Check sheet for the modelled part. Datum: model origin and axes. Units: mm. A direction names the side the tool comes from. Give positions to 0.01 mm unless a question says otherwise; leave off trailing zeros. Loops run counter-clockwise (first coordinate to the right, second up) from the corner with the lowest first, then second, coordinate; pieces in that order, holes last. Notation, with made-up numbers: (28.25, 51.5) - (37.25, 51.5) arc R7 ccw to (37.25, 59.5) - close; hole circle Ø9 at (67.5, -13.75). An arc over 180 degrees is marked (long way). Answer in a Markdown table with one row per item. Add a question column.
(1) Thickness scan on L1, parallel to Z at x = 0.75, y = 2.75; L2, parallel to Z at x = 2.5, y = 2.5; L3, parallel to Z at x = 0.25, y = -2.75. Record the ranges inside material, lowest first.
(2) Sectioned sample at A-A on z = 14. Enter the section's corners in (x, y) (1 decimal), then the cut area to 3 significant figures.
(3) Go/stop test with flat-tipped pins: P1, Ø4, axis at y = -2, z = 27, coming from the +X side; P2, Ø2, axis at x = 3, z = 17, coming from the -Y side; P3, Ø1, axis at x = 0, z = 12, coming from the +Y side; P4, Ø1, axis at y = -4, z = 27, coming from the -X side. Record where each tip stops, or that it passes through.
(4) Sectioned sample at B-B on y = 4.5. Enter the section's corners in (x, z).
(5) Set-up check for faces 1 (the face through (0, 0, 30.607)), 2 (the face through (2, 2, 3.302)): record each of +Z, -Z, +X, -X, +Y, -Y from which the full face is reachable in a straight line by a thin tool's end or side.
from build123d import *

# Parameters (mm, degrees)
SKETCH3_R           = 3.175
BOSS_EXTRUDE1_DEPTH = 3.302
CUT_SWEEP1_PITCH    = 1.27
SKETCH10_R          = 2.2225
BOSS_EXTRUDE5_DEPTH = 26.797
SKETCH9_R           = 5.08
BOSS_EXTRUDE4_DEPTH = 0.127
DOME3_FACE_RADIUS   = 5.08
DOME3_HEIGHT        = 2.38
SKETCH11_R          = 1.8415
BOSS_EXTRUDE6_DEPTH = 0.508


with BuildPart() as part:
    # Sketch3 → Boss-Extrude1 (new body)
    with BuildSketch(Plane.XY):
        with Locations(Location((0, 0, 0), (0, 0, 180))):
            Circle(SKETCH3_R)
    extrude(amount=BOSS_EXTRUDE1_DEPTH)

    # Cut-Sweep1: arcs per turn and ends read off the stored shape
    # Cut-Sweep1: the profile of Sketch5 profile screwed along a left-hand helix through 4.5 turns, 8 arcs to a turn; built about Z, then put on its axis
    cut_sweep1_z = Axis((0, 0, 0), (0, 0, 1))
    cut_sweep1_corners = [(2.54, 0, -1.397), (3.1753, 0, -1.763790626), (3.1753, 0, -0.776209374), (2.54, 0, -1.143)]
    with BuildLine(mode=Mode.PRIVATE) as cut_sweep1_profile:
        Line(cut_sweep1_corners[0], cut_sweep1_corners[1])
        Line(cut_sweep1_corners[1], cut_sweep1_corners[2])
        Line(cut_sweep1_corners[2], cut_sweep1_corners[3])
        Line(cut_sweep1_corners[3], cut_sweep1_corners[0])
    cut_sweep1_cap = Face(cut_sweep1_profile.wire())
    cut_sweep1_turn_angles = [0, -22.5, -45, -67.5, -90, -112.5, -135, -157.5, -180, -202.5, -225, -247.5, -270, -292.5, -315, -337.5, -360]
    cut_sweep1_turn_weights = [1, 0.9238795325112867, 1, 0.9238795325112867, 1, 0.9238795325112867, 1, 0.9238795325112867, 1, 0.9238795325112867, 1, 0.9238795325112867, 1, 0.9238795325112867, 1, 0.9238795325112867, 1]
    cut_sweep1_turn_rails = [Edge.make_bspline([Vector(p[0], p[1], 0).rotate(cut_sweep1_z, cut_sweep1_turn_angles[k]) / cut_sweep1_turn_weights[k] + Vector(0, 0, p[2] + -CUT_SWEEP1_PITCH * cut_sweep1_turn_angles[k] / 360) for k in range(17)], [0, 0, 0, 1, 1, 2, 2, 3, 3, 4, 4, 5, 5, 6, 6, 7, 7, 8, 8, 8], 2, cut_sweep1_turn_weights) for p in cut_sweep1_corners]
    cut_sweep1_turn_sides = [Face.make_surface_from_curves(cut_sweep1_turn_rails[p[0]], cut_sweep1_turn_rails[p[1]]) for p in [(0, 1), (1, 2), (2, 3), (3, 0)]]
    cut_sweep1_last_angles = [-1440, -1462.5, -1485, -1507.5, -1530, -1552.5, -1575, -1597.5, -1620]
    cut_sweep1_last_weights = [1, 0.9238795325112867, 1, 0.9238795325112867, 1, 0.9238795325112867, 1, 0.9238795325112867, 1]
    cut_sweep1_last_rails = [Edge.make_bspline([Vector(p[0], p[1], 0).rotate(cut_sweep1_z, cut_sweep1_last_angles[k]) / cut_sweep1_last_weights[k] + Vector(0, 0, p[2] + -CUT_SWEEP1_PITCH * cut_sweep1_last_angles[k] / 360) for k in range(9)], [0, 0, 0, 1, 1, 2, 2, 3, 3, 4, 4, 4], 2, cut_sweep1_last_weights) for p in cut_sweep1_corners]
    cut_sweep1_last_sides = [Face.make_surface_from_curves(cut_sweep1_last_rails[p[0]], cut_sweep1_last_rails[p[1]]) for p in [(0, 1), (1, 2), (2, 3), (3, 0)]]
    cut_sweep1 = Plane(origin=(0, 0, 0), x_dir=(0, 1, 0), z_dir=(0, 0, 1)) * Solid(Shell([*[p.moved(Location((0, 0, CUT_SWEEP1_PITCH * i))) for i in range(4) for p in cut_sweep1_turn_sides], *cut_sweep1_last_sides, cut_sweep1_cap, cut_sweep1_cap.rotate(cut_sweep1_z, -1620).moved(Location((0, 0, -CUT_SWEEP1_PITCH * -1620 / 360)))]))
    add(cut_sweep1, mode=Mode.SUBTRACT)

    # Sketch10 → Boss-Extrude5 (add)
    with BuildSketch(Plane.XY.offset(3.302)):
        Circle(SKETCH10_R)
    extrude(amount=BOSS_EXTRUDE5_DEPTH)

    # Sketch9 → Boss-Extrude4 (add)
    with BuildSketch(Plane.XY):
        Circle(SKETCH9_R)
    extrude(amount=-BOSS_EXTRUDE4_DEPTH)

    # Dome3: a dome of height H over a round flat face of radius A is a cap of a sphere of radius (A * A + H * H) / (2 * H)
    dome3_r = (DOME3_FACE_RADIUS * DOME3_FACE_RADIUS + DOME3_HEIGHT * DOME3_HEIGHT) / (2 * DOME3_HEIGHT)
    dome3_base = Plane((0, 0, -0.127), z_dir=(0, 0, -1))
    with Locations(dome3_base.offset(DOME3_HEIGHT - dome3_r)):
        dome3_ball = Sphere(dome3_r, mode=Mode.PRIVATE)
    add(split(dome3_ball, bisect_by=dome3_base, keep=Keep.TOP, mode=Mode.PRIVATE))

    # Sketch11 → Boss-Extrude6 (add)
    with BuildSketch(Plane.XY.offset(30.099)):
        Circle(SKETCH11_R)
    extrude(amount=BOSS_EXTRUDE6_DEPTH)


solid = part.part
Reply:
| question | item | result |
|---|---|---|
| 1 | L1 | -1.86 to 0, 0.36 to 1.02, 1.63 to 2.29, 2.9 to 3.3 |
| 1 | L2 | -1.48 to 0 |
| 1 | L3 | -1.9 to 0.36, 0.87 to 1.63, 2.14 to 2.9 |
| 2 | outline | circle Ø4.4 at (0, 0) |
| 2 | area | 15.5 mm^2 |
| 3 | P1 | x = 2.22 |
| 3 | P2 | y = -0.97 |
| 3 | P3 | y = 2.22 |
| 3 | P4 | through |
| 4 | outline | (-2.36, -0.13) arc R4.84 ccw to (2.36, -0.13) - (2.36, 0) - (-2.36, 0) - close |
| 5 | face 1 | +Z, +X, -X, +Y, -Y |
| 5 | face 2 | +Z |
